from build123d import *

# Parameters (mm, degrees)
ESTRUSIONE_ESTRUSIONE1_DEPTH = 2900


with BuildPart() as part:
    # Schizzo1 → Estrusione-Estrusione1 (new body)
    with BuildSketch(Plane.XY):
        with BuildLine():
            ThreePointArc((12.304198043, -5.970812526), (10.731021445, -6.695460987), (10.006372984, -8.268637585))
            Line((10.006372984, -8.268637585), (9.498788398, -8.776222172))
            Line((9.498788398, -8.776222172), (9.498788398, -13.776222172))
            Line((9.498788398, -13.776222172), (11.998788398, -16.276222172))
            Line((11.998788398, -16.276222172), (-10.001211602, -16.276222172))
            Line((-10.001211602, -16.276222172), (-7.501211602, -13.776222172))
            Line((-7.501211602, -13.776222172), (-7.501211602, -8.776222172))
            Line((-7.501211602, -8.776222172), (-8.008796188, -8.268637585))
            ThreePointArc((-8.008796188, -8.268637585), (-8.733444649, -6.695460987), (-10.306621247, -5.970812526))
            Line((-10.306621247, -5.970812526), (-10.501211602, -5.776222172))
            Line((-10.501211602, -5.776222172), (-10.501211602, -2.776222172))
            Line((-10.501211602, -2.776222172), (-10.306621247, -2.581631817))
            ThreePointArc((-10.306621247, -2.581631817), (-8.733444649, -1.856983356), (-8.008796188, -0.283806758))
            Line((-8.008796188, -0.283806758), (-7.501211602, 0.223777828))
            Line((-7.501211602, 0.223777828), (9.498788398, 0.223777828))
            Line((9.498788398, 0.223777828), (10.006372984, -0.283806758))
            ThreePointArc((10.006372984, -0.283806758), (10.731021445, -1.856983356), (12.304198043, -2.581631817))
            Line((12.304198043, -2.581631817), (12.498788398, -2.776222172))
            Line((12.498788398, -2.776222172), (12.498788398, -5.776222172))
            Line((12.498788398, -5.776222172), (12.304198043, -5.970812526))
        make_face()
    extrude(amount=ESTRUSIONE_ESTRUSIONE1_DEPTH)


solid = part.part
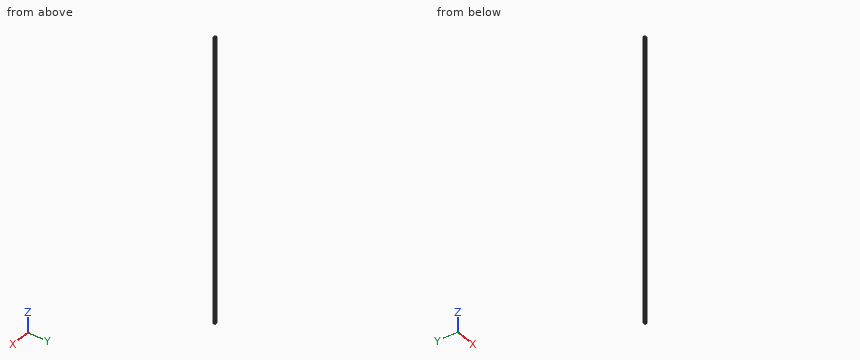
Check sheet for the modelled part. Datum: model origin and axes. Units: mm. Round coordinates to 2 decimals unless told otherwise and drop trailing zeros. Loops run counter-clockwise (first coordinate to the right, second up) from the corner with the lowest first, then second, coordinate; pieces in that order, holes last.
1. Sectioned sample at A-A on z = 2247. Record the boundary of the cut face in (x, y).
2. Gauge pin test, flat ends, axial feed: pin 1 Ø4 at (y, z) = (-10.5, 1187) entering from -X; pin 2 Ø4 at (y, z) = (-11, 1314) entering from +X; pin 3 Ø6 at (y, z) = (-13.5, 2321) entering from +X. Record the tip position at first contact, or that the pin passes through.
3. Scan lines: probe 1 along X at (y, z) = (-9.25, 2012); probe 2 along X at (y, z) = (-14.5, 2254); probe 3 along Y at (x, z) = (10.75, 1009.5). Record each from-to range of solid material in increasing order.
Recorded:
1. outline: (-10.5, -5.78) - (-10.31, -5.97) arc R2.5 cw to (-8.01, -8.27) - (-7.5, -8.78) - (-7.5, -13.78) - (-10, -16.28) - (12, -16.28) - (9.5, -13.78) - (9.5, -8.78) - (10.01, -8.27) arc R2.5 cw to (12.3, -5.97) - (12.5, -5.78) - (12.5, -2.78) - (12.3, -2.58) arc R2.5 cw to (10.01, -0.28) - (9.5, 0.22) - (-7.5, 0.22) - (-8.01, -0.28) arc R2.5 cw to (-10.31, -2.58) - (-10.5, -2.78) - close
2. pin 1: stops at x = -7.78
2. pin 2: stops at x = 9.5
2. pin 3: stops at x = 12
3. probe 1: x = -7.5 to 9.5
3. probe 2: x = -8.22 to 10.22
3. probe 3: y = -16.28 to -15.03, -6.68 to -1.88
